Check sheet for the modelled part. Datum: model origin and axes. Units: mm. A direction names the side the tool comes from. Give positions to 0.01 mm unless a question says otherwise; leave off trailing zeros. Order: outer loops, then holes, each group sorted by start corner. A loop starts at its lowest first (then second) coordinate and runs counter-clockwise, first axis right, second up.
Item 1: Access from +Z, -Z, +X, -X, +Y, -Y to the whole of each face (thin tool, end or side, straight path). Record for faces 4 (the flat face through (0, 3, 2)), 5 (the conical face through (-0.02, 1.24, 1.87)), 6 (the flat face through (-3, 0, 2)), 7 (the flat face through (3, 0, 2)).
Item 2: Sectioned sample at A-A on y = -5.75. Record the boundary of the cut face in (x, z), and give its area (3 significant figures).
Item 3: Release check for a two-part mould opening along Y. For faces 1 (the cylindrical face through (5.155, -6.206, 0.493)), 2 (the flat face through (-2.2, 0, 3)), 3 (the flat face through (0, -3, 2)) record: released by +Y, released by -Y, zero draft, split by the parting line, or undercut.
Item 4: Sectioned sample at C-C on x = 3.75. Record the boundary of the cut face in (y, z).
Item 5: Material ranges on line 1 along Y through (x, z) = (-5.75, 0.4); line 2 along Z through (x, y) = (6, 4.25); line 3 along Y through (x, z) = (-2.5, 2.4), recorded low to high.
Item 6: Gauge pin test, flat ends, axial feed: P1, Ø2.5, axis at x = 5.75, y = 5.75, coming from the +Z side; P2, Ø0.6, axis at x = -1.5, z = 1.5, coming from the +Y side; P3, Ø6, axis at x = 0.5, y = -0.5, coming from the +Z side; P4, Ø1.6, axis at y = -0.5, z = 2, coming from the -X side. Record the tip position at first contact, or that the pin passes through.
Item 7: Sectioned sample at B-B on z = 0.3. Record the boundary of the cut face in (x, y).
from build123d import *

# Parameters (mm, degrees)
F2_DEPTH  = 3
F0_W      = 0.3
F0_H      = 4
F3_DEPTH  = 3
F4_DEPTH  = 3
F7_DEPTH  = 3
F8_DEPTH  = 2
F9_DEPTH  = 1
F11_DEPTH = 3
F12_DEPTH = 2
F13_DEPTH = 1
F15_DEPTH = 1
F16_DEPTH = 1
F0_R      = 0.75
F17_DEPTH = 1


with BuildPart() as f2:
    # F0 (on Top) → F2 (new body)
    with BuildSketch(Plane.XY):
        Polygon((-0.6, -2), (-2, 0), (-2, -2), align=None)
    extrude(amount=F2_DEPTH)


with BuildPart() as f2b:
    # F0 (on Top) → F2, piece 2 (new body)
    with BuildSketch(Plane.XY):
        Polygon((-0.6, 2), (-2, 2), (-2, 0), align=None)
    extrude(amount=F2_DEPTH)


with BuildPart() as f2c:
    # F0 (on Top) → F2, piece 3 (new body)
    with BuildSketch(Plane.XY):
        Polygon((2, 2), (0.6, 2), (2, 0), align=None)
    extrude(amount=F2_DEPTH)


with BuildPart() as f2d:
    # F0 (on Top) → F2, piece 4 (new body)
    with BuildSketch(Plane.XY):
        Polygon((2, -2), (2, 0), (0.6, -2), align=None)
    extrude(amount=F2_DEPTH)


with BuildPart() as f3:
    # F0 (on Top) → F3 (new body)
    with BuildSketch(Plane.XY):
        Polygon((-0.6, -2), (-0.6, 2), (-2, 0), align=None)
        with Locations((-0.45, 0)):
            Rectangle(F0_W, F0_H)
        with Locations((-0.15, 0)):
            Rectangle(F0_W, F0_H)
    extrude(amount=F3_DEPTH)


with BuildPart() as f4:
    # F0 (on Top) → F4 (new body)
    with BuildSketch(Plane.XY):
        with Locations((0.45, 0)):
            Rectangle(F0_W, F0_H)
        Polygon((2, 0), (0.6, 2), (0.6, -2), align=None)
        with Locations((0.15, 0)):
            Rectangle(F0_W, F0_H)
    extrude(amount=F4_DEPTH)


with BuildPart() as f5_tool:
    # F4_face (on face) → F5 (revolve)
    with BuildSketch(Plane(origin=(0.7128205128, 0, 3), x_dir=(1, 0, 0), z_dir=(0, 0, 1))):
        Polygon((-0.1128205128, -2), (1.2871794872, 0), (-0.1128205128, 2), (-0.7128205128, 2), (-0.7128205128, -2), align=None)
    revolve(axis=Axis((0, 0, 3), (0, -1, 0)))


with BuildPart() as f3_1:
    add(f3.part)

    # F5: cut by f5_tool
    add(f5_tool.part, mode=Mode.SUBTRACT)


with BuildPart() as f4_1:
    add(f4.part)

    # F5: cut by f5_tool
    add(f5_tool.part, mode=Mode.SUBTRACT)


with BuildPart() as f2b_1:
    add(f2b.part)

    # F6: union F2, F3, F4, F2c, F2d
    add(f2.part)
    add(f3_1.part)
    add(f4_1.part)
    add(f2c.part)
    add(f2d.part)


with BuildPart() as f7:
    # F1 (on Front) → F7 (new body)
    with BuildSketch(Plane.XZ):
        with BuildLine():
            ThreePointArc((-0.6, 3), (-0.4242640687, 2.5757359313), (0, 2.4))
            Line((0, 2.4), (0, 2.7))
            ThreePointArc((0, 2.7), (-0.2121320344, 2.7878679656), (-0.3, 3))
            Line((-0.3, 3), (-0.6, 3))
        make_face()
        with BuildLine():
            Line((0, 2.7), (0, 2.4))
            ThreePointArc((0, 2.4), (0.4242640687, 2.5757359313), (0.6, 3))
            Line((0.6, 3), (0.3, 3))
            ThreePointArc((0.3, 3), (0.2121320344, 2.7878679656), (0, 2.7))
        make_face()
    extrude(amount=F7_DEPTH)

    # F1 (on Front) → F8 (cut)
    with BuildSketch(Plane.XZ):
        with BuildLine():
            ThreePointArc((-0.6, 3), (-0.4242640687, 2.5757359313), (0, 2.4))
            Line((0, 2.4), (0, 2.7))
            ThreePointArc((0, 2.7), (-0.2121320344, 2.7878679656), (-0.3, 3))
            Line((-0.3, 3), (-0.6, 3))
        make_face()
        with BuildLine():
            Line((0, 2.7), (0, 2.4))
            ThreePointArc((0, 2.4), (0.4242640687, 2.5757359313), (0.6, 3))
            Line((0.6, 3), (0.3, 3))
            ThreePointArc((0.3, 3), (0.2121320344, 2.7878679656), (0, 2.7))
        make_face()
    extrude(amount=F8_DEPTH, mode=Mode.SUBTRACT)


with BuildPart() as f9:
    # F9 (new): a face of the model
    f9_faces = [f2b_1.part.faces().sort_by_distance(p)[0] for p in [
        (0, -2, 1.4384118942),
    ]]
    extrude(f9_faces, amount=F9_DEPTH)


with BuildPart() as f7_1:
    add(f7.part)

    # F10: union F2b, F9
    add(f2b_1.part)
    add(f9.part)


with BuildPart() as f11:
    # F1 (on Front) → F11 (new body)
    with BuildSketch(Plane.XZ):
        with BuildLine():
            Line((0, 2.7), (0, 2.4))
            ThreePointArc((0, 2.4), (0.4242640687, 2.5757359313), (0.6, 3))
            Line((0.6, 3), (0.3, 3))
            ThreePointArc((0.3, 3), (0.2121320344, 2.7878679656), (0, 2.7))
        make_face()
        with BuildLine():
            ThreePointArc((-0.6, 3), (-0.4242640687, 2.5757359313), (0, 2.4))
            Line((0, 2.4), (0, 2.7))
            ThreePointArc((0, 2.7), (-0.2121320344, 2.7878679656), (-0.3, 3))
            Line((-0.3, 3), (-0.6, 3))
        make_face()
    extrude(amount=-F11_DEPTH)

    # F1 (on Front) → F12 (cut)
    with BuildSketch(Plane.XZ):
        with BuildLine():
            Line((0, 2.7), (0, 2.4))
            ThreePointArc((0, 2.4), (0.4242640687, 2.5757359313), (0.6, 3))
            Line((0.6, 3), (0.3, 3))
            ThreePointArc((0.3, 3), (0.2121320344, 2.7878679656), (0, 2.7))
        make_face()
        with BuildLine():
            ThreePointArc((-0.6, 3), (-0.4242640687, 2.5757359313), (0, 2.4))
            Line((0, 2.4), (0, 2.7))
            ThreePointArc((0, 2.7), (-0.2121320344, 2.7878679656), (-0.3, 3))
            Line((-0.3, 3), (-0.6, 3))
        make_face()
    extrude(amount=-F12_DEPTH, mode=Mode.SUBTRACT)


with BuildPart() as f13:
    # F13 (new): a face of the model
    f13_faces = [f7_1.part.faces().sort_by_distance(p)[0] for p in [
        (0, 2, 1.4384118942),
    ]]
    extrude(f13_faces, amount=F13_DEPTH)


with BuildPart() as f11_1:
    add(f11.part)

    # F14: union F13, F7
    add(f13.part)
    add(f7_1.part)

    # F15 (add): a face of the model
    f15_faces = [f11_1.faces().sort_by_distance(p)[0] for p in [
        (2, 0, 1.5),
    ]]
    extrude(f15_faces, amount=F15_DEPTH)

    # F16 (add): a face of the model
    f16_faces = [f11_1.faces().sort_by_distance(p)[0] for p in [
        (-2, 0, 1.5),
    ]]
    extrude(f16_faces, amount=F16_DEPTH)

    # F0 (on Top) → F17 (join)
    with BuildSketch(Plane.XY):
        Polygon((9.5, 9.5), (-6.5961940777, 9.5), (-9.5, 6.5961940777), (-9.5, -9.5), (9.5, -9.5), align=None)
        with Locations((-5.75, -5.75)):
            Circle(F0_R, mode=Mode.SUBTRACT)
        with Locations((5.75, -5.75)):
            Circle(F0_R, mode=Mode.SUBTRACT)
        with Locations((-5.75, 5.75)):
            Circle(F0_R, mode=Mode.SUBTRACT)
        Polygon((-2, 0), (-2, 2), (-0.6, 2), (-0.3, 2), (0, 2), (0.3, 2), (0.6, 2), (2, 2), (2, 0), (2, -2), (0.6, -2), (0.3, -2), (0, -2), (-0.3, -2), (-0.6, -2), (-2, -2), align=None, mode=Mode.SUBTRACT)
        with Locations((5.75, 5.75)):
            Circle(F0_R, mode=Mode.SUBTRACT)
    extrude(amount=F17_DEPTH)


solid = f11_1.part
Report:
1. face 4: +Z, +X, -X, +Y
1. face 5: +Z
1. face 6: +Z, -X, +Y, -Y
1. face 7: +Z, +X, +Y, -Y
2. outline: (-9.5, 0) - (-6.5, 0) - (-6.5, 1) - (-9.5, 1) - close; (-5, 0) - (5, 0) - (5, 1) - (-5, 1) - close; (6.5, 0) - (9.5, 0) - (9.5, 1) - (6.5, 1) - close
2. area: 16.0 mm2
3. face 1: undercut
3. face 2: zero draft
3. face 3: released by -Y
4. outline: (-9.5, 0) - (9.5, 0) - (9.5, 1) - (-9.5, 1) - close
5. line 1: y = -9.5 to -6.5, -5 to 5, 6.5 to 9.5
5. line 2: z = 0 to 1
5. line 3: y = -3 to 3
6. P1: stops at z = 1
6. P2: stops at y = 3
6. P3: stops at z = 3
6. P4: stops at x = -3
7. outline: (-9.5, -9.5) - (9.5, -9.5) - (9.5, 9.5) - (-6.6, 9.5) - (-9.5, 6.6) - close; hole circle Ø1.5 at (-5.75, -5.75); hole circle Ø1.5 at (-5.75, 5.75); hole circle Ø1.5 at (5.75, -5.75); hole circle Ø1.5 at (5.75, 5.75)
